from build123d import *

# Parameters (mm, degrees)
F0_W     = 600
F0_H     = 194
F0_R     = 3.25
F1_DEPTH = 8
F2_W     = 600
F2_H     = 194
F2_W_2   = 564
F2_H_2   = 158
F3_DEPTH = 2
F4_SIZE  = 0.5
F5_R     = 2.5
F6_DEPTH = 25
F7_SIZE  = 0.5


with BuildPart() as f1:
    # F0 (on Top) → F1 (new body)
    with BuildSketch(Plane.XY):
        Rectangle(F0_W, F0_H)
        with Locations((-250, -88)):
            Circle(F0_R, mode=Mode.SUBTRACT)
        with Locations((-291, -70)):
            Circle(F0_R, mode=Mode.SUBTRACT)
        with Locations((-125, -88)):
            Circle(F0_R, mode=Mode.SUBTRACT)
        with Locations((0, -88)):
            Circle(F0_R, mode=Mode.SUBTRACT)
        with Locations((125, -88)):
            Circle(F0_R, mode=Mode.SUBTRACT)
        with Locations((250, -88)):
            Circle(F0_R, mode=Mode.SUBTRACT)
        with Locations((291, -70)):
            Circle(F0_R, mode=Mode.SUBTRACT)
        with Locations((-291, 0)):
            Circle(F0_R, mode=Mode.SUBTRACT)
        with Locations((-291, 70)):
            Circle(F0_R, mode=Mode.SUBTRACT)
        with Locations((-250, 88)):
            Circle(F0_R, mode=Mode.SUBTRACT)
        with Locations((-125, 88)):
            Circle(F0_R, mode=Mode.SUBTRACT)
        with Locations((291, 0)):
            Circle(F0_R, mode=Mode.SUBTRACT)
        with Locations((0, 88)):
            Circle(F0_R, mode=Mode.SUBTRACT)
        with Locations((125, 88)):
            Circle(F0_R, mode=Mode.SUBTRACT)
        with Locations((291, 70)):
            Circle(F0_R, mode=Mode.SUBTRACT)
        with Locations((250, 88)):
            Circle(F0_R, mode=Mode.SUBTRACT)
    extrude(amount=F1_DEPTH)

    # F2 (on face) → F3 (cut)
    with BuildSketch(Plane.XY.offset(8)):
        Rectangle(F2_W, F2_H)
        Rectangle(F2_W_2, F2_H_2, mode=Mode.SUBTRACT)
    extrude(amount=-F3_DEPTH, mode=Mode.SUBTRACT)

    # F4
    f4_edges = [f1.edges().sort_by_distance(p)[0] for p in [
        (-294.25, 70, 0),
        (-287.75, 70, 3),
        (-294.25, 70, 6),
        (-294.25, 0, 0),
        (-287.75, 0, 3),
        (-294.25, 0, 6),
        (-253.25, 88, 0),
        (-246.75, 88, 3),
        (-253.25, 88, 6),
        (-294.25, -70, 0),
        (-287.75, -70, 3),
        (-294.25, -70, 6),
        (-253.25, -88, 0),
        (-246.75, -88, 3),
        (-253.25, -88, 6),
        (-128.25, -88, 0),
        (-121.75, -88, 3),
        (-128.25, -88, 6),
        (-3.25, -88, 0),
        (3.25, -88, 3),
        (-3.25, -88, 6),
        (121.75, -88, 0),
        (128.25, -88, 3),
        (121.75, -88, 6),
        (246.75, -88, 0),
        (253.25, -88, 3),
        (246.75, -88, 6),
        (287.75, -70, 0),
        (294.25, -70, 3),
        (287.75, -70, 6),
        (287.75, 70, 0),
        (294.25, 70, 3),
        (287.75, 70, 6),
        (246.75, 88, 0),
        (253.25, 88, 3),
        (246.75, 88, 6),
        (121.75, 88, 0),
        (128.25, 88, 3),
        (121.75, 88, 6),
        (-3.25, 88, 0),
        (3.25, 88, 3),
        (-3.25, 88, 6),
        (-128.25, 88, 0),
        (-121.75, 88, 3),
        (-128.25, 88, 6),
        (287.75, 0, 0),
        (294.25, 0, 3),
        (287.75, 0, 6),
    ]]
    chamfer(f4_edges, length=F4_SIZE)

    # F5 (on face) → F6 (cut)
    with BuildSketch(Plane.XY.offset(8)):
        with Locations((-222.5, 69)):
            Circle(F5_R)
        with Locations((222.5, 69)):
            Circle(F5_R)
    extrude(amount=-F6_DEPTH, mode=Mode.SUBTRACT)

    # F7
    f7_edges = [f1.edges().sort_by_distance(p)[0] for p in [
        (-225, 69, 8),
        (-220, 69, 4),
        (-225, 69, 0),
        (220, 69, 8),
        (225, 69, 4),
        (220, 69, 0),
    ]]
    chamfer(f7_edges, length=F7_SIZE)


solid = f1.part
Input: part model. Units: mm. Frame: model coordinates. Round coordinates to 2 decimals unless told otherwise and drop trailing zeros. Order: outer loops, then holes, each group sorted by start corner. A loop starts at its lowest first (then second) coordinate and runs counter-clockwise, first axis right, second up. Notation, with made-up numbers: (36, 22) - (61, 22) arc R27 ccw to (61, 43) - close; hole circle Ø2 at (59.5, 68). An arc over 180 degrees is marked (long way). Answer as a JSON object with one key per item and string values. Group by question number.
(1) Cut plane B-B (x = 10.5). Return loops of the section in (y, z), then the cut area to 3 significant figures.
(2) Material intervals for probe 1 along Y at (x, z) = (-125, 4); probe 2 along Y at (x, z) = (291, 2); probe 3 along X at (y, z) = (88, 4.45), sorted ascending. Write a range as from..to.
(3) Cut plane A-A (y = 53). Return loops of the section in (x, z).
(4) Pin query (flat end, axial travel): P1, Ø0.6, axis at x = -136.5, z = 7, coming from the +Y side; P2, Ø1.6, axis at y = -25, z = 7.5, coming from the -X side; P3, Ø8.5, axis at x = -250, y = -88, coming from the +Z side. Return the tip coordinate at first contact, or that it passes through.
(5) Draft query along Z for faces 1 (the face through (-1.4, 79.5, 6)), 2 (the face through (-4, 1, 0)). Return one class per face: released by +Z, released by -Z, zero draft, split by the parting line, or undercut.
Here are the results:
{
 "1": {"outline": "(-97, 0) - (97, 0) - (97, 6) - (79, 6) - (79, 8) - (-79, 8) - (-79, 6) - (-97, 6) - close", "area": "1,480 mm^2"},
 "2": {"probe 1": "y = -97..-91.25, -84.75..84.75, 91.25..97", "probe 2": "y = -97..-73.25, -66.75..-3.25, 3.25..66.75, 73.25..97", "probe 3": "x = -300..-253.25, -246.75..-128.25, -121.75..-3.25, 3.25..121.75, 128.25..246.75, 253.25..300"},
 "3": {"outline": "(-300, 0) - (300, 0) - (300, 6) - (282, 6) - (282, 8) - (-282, 8) - (-282, 6) - (-300, 6) - close"},
 "4": {"P1": "stops at y = 79", "P2": "stops at x = -282", "P3": "stops at z = 6"},
 "5": {"face 1": "released by +Z", "face 2": "released by -Z"}
}
